Input: part model. Units: mm. Frame: model coordinates. Coordinates: 2 decimals unless noted, no trailing zeros. Loops run counter-clockwise (first coordinate to the right, second up) from the corner with the lowest first, then second, coordinate; pieces in that order, holes last. Notation, with made-up numbers: (-25.5, 56) -> (14.5, 56) arc R22 ccw to (14.5, 93) -> close; hole circle Ø11 at (50, -28). An arc over 180 degrees is marked (long way). Answer as a JSON object with one key per item and string values.
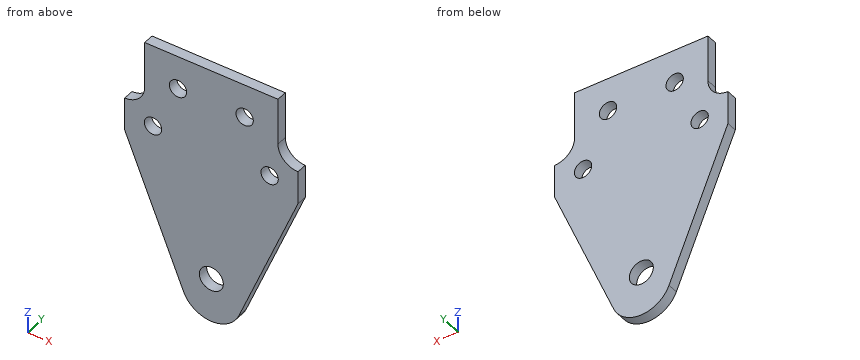
from build123d import *

# Parameters (mm, degrees)
SKETCH1_R           = 2.6
SKETCH1_R_2         = 3.6
BOSS_EXTRUDE1_DEPTH = 3.175


with BuildPart() as part:
    # Sketch1 → Boss-Extrude1 (new body)
    with BuildSketch(Plane(origin=(0, 0, 0), x_dir=(1, 0, 0), z_dir=(0, 1, 0))):
        with BuildLine():
            Line((8.314915793, 72.695604767), (26, 30.000034622))
            Line((26, 30.000034622), (26, 20.000034622))
            ThreePointArc((26, 20.000034622), (21.757357213, 18.242652928), (20, 14))
            Line((20, 14), (20, 0))
            Line((20, 0), (-20, 0))
            Line((-20, 0), (-20, 14))
            ThreePointArc((-20, 14), (-21.757357213, 18.242652928), (-26, 20.000034622))
            Line((-26, 20.000034622), (-26, 30.000034622))
            Line((-26, 30.000034622), (-8.314915793, 72.695604767))
            ThreePointArc((-8.314915793, 72.695604767), (0, 78.251453876), (8.314915793, 72.695604767))
        make_face()
        with Locations((10, 10)):
            Circle(SKETCH1_R, mode=Mode.SUBTRACT)
        with Locations((-17.5, 25)):
            Circle(SKETCH1_R, mode=Mode.SUBTRACT)
        with Locations((0, 65)):
            Circle(SKETCH1_R_2, mode=Mode.SUBTRACT)
        with Locations((17.5, 25)):
            Circle(SKETCH1_R, mode=Mode.SUBTRACT)
        with Locations((-10, 10)):
            Circle(SKETCH1_R, mode=Mode.SUBTRACT)
    extrude(amount=BOSS_EXTRUDE1_DEPTH)


solid = part.part
1. Pin query (flat end, axial travel): P1, Ø1, axis at y = 2, z = -39.5, coming from the -X side; P2, Ø1.6, axis at y = 2, z = -7, coming from the +X side; P3, Ø1.5, axis at y = 2, z = -51, coming from the -X side. Return the tip coordinate at first contact, or that it passes through.
Reply:
{"P1": "stops at x = -22.27", "P2": "stops at x = 20", "P3": "stops at x = -17.61"}
2. Section query B-B (y = 2.65). Return loops of the section in (x, z), plus the area to 3 significant figures.
Reply:
{"outline": "(-26, -30) -> (-8.31, -72.7) arc R9 ccw to (8.31, -72.7) -> (26, -30) -> (26, -20) arc R6 cw to (20, -14) -> (20, 0) -> (-20, 0) -> (-20, -14) arc R6 cw to (-26, -20) -> close; hole circle Ø5.2 at (-17.5, -25); hole circle Ø5.2 at (-10, -10); hole circle Ø7.2 at (0, -65); hole circle Ø5.2 at (10, -10); hole circle Ø5.2 at (17.5, -25)", "area": "2,740 mm2"}
3. Section query A-A (x = 0). Return loops of the section in (y, z) (3 decimals), plus the area to 3 significant figures.
Reply:
{"outline": "(0, -78.251) -> (3.175, -78.251) -> (3.175, -68.6) -> (0, -68.6) -> close; (0, -61.4) -> (3.175, -61.4) -> (3.175, 0) -> (0, 0) -> close", "area": "226 mm2"}
4. Line query: line 1 along X through (y, z) = (1.9, -10); line 2 along X through (y, z) = (2.45, -25); line 3 along Z through (x, y) = (0, 2.5). Output: solid intervals per line, ascending.
Reply:
{"line 1": "x = -20 to -12.6, -7.4 to 7.4, 12.6 to 20", "line 2": "x = -26 to -20.1, -14.9 to 14.9, 20.1 to 26", "line 3": "z = -78.25 to -68.6, -61.4 to 0"}
5. Section query C-C (z = -65). Return loops of the section in (x, y) (3 decimals).
Reply:
{"outline": "(-11.503, 0) -> (-3.6, 0) -> (-3.6, 3.175) -> (-11.503, 3.175) -> close; (3.6, 0) -> (11.503, 0) -> (11.503, 3.175) -> (3.6, 3.175) -> close"}
6. Section query D-D (z = -19). Return loops of the section in (x, y) (3 decimals).
Reply:
{"outline": "(-22.683, 0) -> (22.683, 0) -> (22.683, 3.175) -> (-22.683, 3.175) -> close"}
